```python
from build123d import *

# Parameters (mm, degrees)
SKETCH2_R          = 29
SKETCH2_R_2        = 25
SKETCH3_R          = 27
SKETCH3_R_2        = 25
CUT_EXTRUDE1_DEPTH = 7
SKETCH8_R          = 29
SKETCH8_R_2        = 22
CUT_EXTRUDE3_DEPTH = 4


with BuildPart() as part:
    # Sweep1: sweep along a path in Sketch1
    with BuildLine(Plane.XY) as sweep1_path:
        Line((-20, 30), (0, 30))
        ThreePointArc((0, 30), (21.213203436, 21.213203436), (30, 0))
        Line((30, 0), (30, -33))
    # Sketch2 → Sweep1 (sweep)
    with BuildSketch(Plane(origin=(0, -33, 0), x_dir=(1, 0, 0), z_dir=(0, 1, 0))):
        with Locations((30, 0)):
            Circle(SKETCH2_R)
        with Locations((30, 0)):
            Circle(SKETCH2_R_2, mode=Mode.SUBTRACT)
    sweep(path=sweep1_path.line)

    # Sketch3 → Cut-Extrude1 (cut)
    with BuildSketch(Plane.ZY.offset(20)):
        with Locations((0, 30)):
            Circle(SKETCH3_R)
        with Locations((0, 30)):
            Circle(SKETCH3_R_2, mode=Mode.SUBTRACT)
    extrude(amount=-CUT_EXTRUDE1_DEPTH, mode=Mode.SUBTRACT)

    # Sketch7 → Revolve2 (revolve)
    with BuildSketch(Plane(origin=(30, 0, 0), x_dir=(0, 0, -1), z_dir=(1, 0, 0))):
        Polygon((25, 0), (20, -33), (25, -33), align=None)
    revolve(axis=Axis((30, 0, 0), (0, -1, 0)))

    # Sketch8 → Cut-Extrude3 (cut)
    with BuildSketch(Plane.XZ.offset(33)):
        with Locations((30, 0)):
            Circle(SKETCH8_R)
        with Locations((30, 0)):
            Circle(SKETCH8_R_2, mode=Mode.SUBTRACT)
    extrude(amount=-CUT_EXTRUDE3_DEPTH, mode=Mode.SUBTRACT)

    # Sketch10 → Cut-Revolve2 (revolve, cut)
    with BuildSketch(Plane(origin=(30, 0, 0), x_dir=(0, 0, -1), z_dir=(1, 0, 0))):
        Polygon((29, 0), (25, -29), (29, -29), align=None)
    revolve(axis=Axis((30, 0, 0), (0, -1, 0)), mode=Mode.SUBTRACT)


solid = part.part
```
The model under review builds one solid part; all positions refer to its coordinate system, in mm. A direction names the side the tool comes from. Round coordinates to 2 decimals unless told otherwise and drop trailing zeros. Order: outer loops, then holes, each group sorted by start corner. A loop starts at its lowest first (then second) coordinate and runs counter-clockwise, first axis right, second up. Notation, with made-up numbers: (84, 47.5) -> (107, 47.5) arc R22 cw to (107, 65.5) -> close; hole circle Ø11 at (46.5, -39.75). An arc over 180 degrees is marked (long way). Use a Markdown table: item, result.
Q1. Tool access review of faces 4 (the conical face through (8.6, -20.4, 4.7)), 5 (the flat face through (12, -33, 10)), 6 (the cylindrical face through (25.231, -31.028, -21.477)), 7 (the cylindrical face through (-16.55, 56.77, -3.51)): name each direction out of +Z, -Z, +X, -X, +Y, -Y from which nothing blocks a thin tool from reaching the whole face with its end or side.
Values:
| item | result |
|---|---|
| face 4 | none |
| face 5 | +Z, -Z, +X, -X, -Y |
| face 6 | -Y |
| face 7 | -X |
Q2. We need section C-C on y = -7.5. Write out the cut boundary in (x, z), then the cut area to 3 significant figures.
Values:
| item | result |
|---|---|
| outline | circle Ø55.93 at (30, 0); hole circle Ø47.73 at (30, 0) |
| area | 668 mm^2 |
Q3. Mouldability with a two-part tool opening along Y and no side actions: class faces 1 (the cylindrical face through (-6.409, 53.846, 7.509)), 2 (the flat face through (31.7, -29, -22.1)), 3 (the cylindrical face through (-9.86, 6.99, -17.65)) as +Y half, -Y half, draft (parallel to the pull), parting line (faces both ways), or undercut.
Values:
| item | result |
|---|---|
| face 1 | undercut |
| face 2 | -Y half |
| face 3 | parting line |
Q4. For line 1 (Z direction, x = 25, y = -23); line 2 (Z direction, x = 30.5, y = 22.5); line 3 (Y direction, x = -7.5, z = -0.5) (3 decimals), list the stretches that pass through material, from the lowest coordinate up.
Values:
| item | result |
|---|---|
| line 1 | z = -25.34 to -20.93, 20.93 to 25.34 |
| line 2 | z = -27.9 to -23.72, 23.72 to 27.9 |
| line 3 | y = 1.004 to 5.005, 54.995 to 58.996 |
Q5. Clearance check with flat-ended pins moving along their axes: P1, Ø8, axis at x = -9.5, z = 17.5, coming from the -Y side; P2, Ø6, axis at y = -10.5, z = 9.5, coming from the -X side; P3, Ø2, axis at y = -5, z = 12, coming from the -X side. State where each tip first meets the part, or that it passes through.
Values:
| item | result |
|---|---|
| P1 | stops at y = 4.33 |
| P2 | stops at x = 3.11 |
| P3 | stops at x = 3.89 |
Q6. We need section A-A on z = 0. Write out the cut boundary in (x, y).
Values:
| item | result |
|---|---|
| outline | (-20, 1) -> (0, 1) arc R1 cw to (1, 0) -> (5, -29) -> (8, -29) -> (8, -33) -> (10, -33) -> (5, 0) arc R5 ccw to (0, 5) -> (-13, 5) -> (-13, 3) -> (-20, 3) -> close; (-20, 57) -> (-13, 57) -> (-13, 55) -> (0, 55) arc R55 cw to (55, 0) -> (50, -33) -> (52, -33) -> (52, -29) -> (55, -29) -> (59, 0) arc R59 ccw to (0, 59) -> (-20, 59) -> close |
Q7. We need section B-B on x = -11. Write out the cut boundary in (y, z).
Values:
| item | result |
|---|---|
| outline | circle Ø58 at (30, 0); hole circle Ø50 at (30, 0) |
